Input: part model. Units: mm. Frame: model coordinates. Coordinates: 2 decimals unless noted, no trailing zeros. Order: outer loops, then holes, each group sorted by start corner. A loop starts at its lowest first (then second) coordinate and runs counter-clockwise, first axis right, second up. Notation, with made-up numbers: (-23.5, 46) -> (33.5, 46) arc R13 ccw to (33.5, 57) -> close; hole circle Ø8 at (70.25, 50.25). An arc over 180 degrees is marked (long way). Write each question's results on one line, items separated by ' | '.
```python
from build123d import *

# Parameters (mm, degrees)
SKETCH1_R           = 1.5
BOSS_EXTRUDE1_DEPTH = 1.35
CHAMFER1_SIZE       = 0.4


with BuildPart() as part:
    # Sketch1 → Boss-Extrude1 (new, symmetric)
    with BuildSketch(Plane(origin=(0, 0, 0), x_dir=(1, 0, 0), z_dir=(0, 1, 0))):
        with BuildLine():
            Line((-13, 3.5), (13, 3.5))
            ThreePointArc((13, 3.5), (16.5, 0), (13, -3.5))
            Line((13, -3.5), (-13, -3.5))
            ThreePointArc((-13, -3.5), (-16.5, 0), (-13, 3.5))
        make_face()
        with Locations(Location((-13, 0, 0), (0, 0, 90))):
            Circle(SKETCH1_R, mode=Mode.SUBTRACT)
        with Locations(Location((13, 0, 0), (0, 0, 90))):
            Circle(SKETCH1_R, mode=Mode.SUBTRACT)
    extrude(amount=BOSS_EXTRUDE1_DEPTH, both=True)

    # Chamfer1
    chamfer1_edges = [part.edges().sort_by_distance(p)[0] for p in [
        (16.5, 1.35, 0),
        (0, 1.35, -3.5),
        (-16.5, 1.35, 0),
        (0, 1.35, 3.5),
    ]]
    chamfer(chamfer1_edges, length=CHAMFER1_SIZE)


solid = part.part
```
(1) Pin query (flat end, axial travel): P1, Ø2.5, axis at x = -13, z = 0, coming from the +Y side; P2, Ø1.5, axis at y = 0, z = -2, coming from the -X side. Return the tip coordinate at first contact, or that it passes through.
Return value:
P1: through | P2: x = -16.27
(2) Cut plane B-B, the plane y = 0.05. Return loops of the section in (x, z), plus the area to 3 significant figures.
Return value:
outline: (-13, -3.5) -> (13, -3.5) arc R3.5 ccw to (13, 3.5) -> (-13, 3.5) arc R3.5 ccw to start; hole circle Ø3 at (-13, 0); hole circle Ø3 at (13, 0) | area: 206 mm2
(3) Line query: line 1 along X through (y, z) = (-0.3, 0); line 2 along Z through (x, y) = (-13, 0); line 3 along X through (y, z) = (-0.75, -0.5). Output: solid intervals per line, ascending. Write a range as from..to.
Return value:
line 1: -16.5..-14.5, -11.5..11.5, 14.5..16.5 | line 2: -3.5..-1.5, 1.5..3.5 | line 3: -16.46..-14.41, -11.59..11.59, 14.41..16.46
(4) Cut plane A-A, the plane z = 0. Return loops of the section in (x, y).
Return value:
outline: (-16.5, -1.35) -> (-14.5, -1.35) -> (-14.5, 1.35) -> (-16.1, 1.35) -> (-16.5, 0.95) -> close; (-11.5, -1.35) -> (11.5, -1.35) -> (11.5, 1.35) -> (-11.5, 1.35) -> close; (14.5, -1.35) -> (16.5, -1.35) -> (16.5, 0.95) -> (16.1, 1.35) -> (14.5, 1.35) -> close
(5) Mould query, pull axis Z, two halves, no side actions, for faces 1 (the face through (12.55, -0.02, -1.43)), 2 (the face through (-16.5, -0.2, 0.1)), 3 (the face through (0, 0, 3.5)). Classes: +Z half, -Z half, draft (parallel to the pull), parting line (faces both ways), or undercut.
Return value:
face 1: undercut | face 2: parting line | face 3: +Z half
